```python
from build123d import *

# Parameters (mm, degrees)
BOSS_EXTRUDE1_DEPTH   = 40
BOSS_EXTRUDE1_2_DEPTH = 40
BOSS_EXTRUDE2_DEPTH   = 5


with BuildPart() as part:
    # Sketch2 → Boss-Extrude1 (new body)
    with BuildSketch(Plane.XY.offset(-35)):
        Polygon((-29.235736387, -93.619070837), (-29.235736387, -98.170199329), (-20.059825436, -100.584912737), (-20.059825436, -93.619070837), align=None)
    extrude(amount=BOSS_EXTRUDE1_DEPTH)



with BuildPart() as body_2:
    # Sketch2 → Boss-Extrude1 2 (new body)
    with BuildSketch(Plane.XY.offset(-35)):
        Polygon((29.235736387, -98.170199329), (20.059825436, -100.584912737), (20.059825436, -93.619070837), (29.235736387, -93.619070837), align=None)
    extrude(amount=BOSS_EXTRUDE1_2_DEPTH)


with BuildPart() as part_1:
    add(part.part)

    add(body_2.part)  # Boss-Extrude2 merges body 2
    # Sketch3 → Boss-Extrude2 (add)
    with BuildSketch(Plane.XY):
        Polygon((-46.530024654, -93.619070837), (0.133009642, -93.619070837), (46.530024654, -93.619070837), (46.530024654, -95.999382249), (0.133009642, -107.832641703), (-46.530024654, -95.999382249), align=None)
    extrude(amount=BOSS_EXTRUDE2_DEPTH)


solid = part_1.part
```
Geometry check sheet. Reference: the model listing, model coordinates, mm. A direction names the side the tool comes from. Round coordinates to 2 decimals unless told otherwise and drop trailing zeros. Loops run counter-clockwise (first coordinate to the right, second up) from the corner with the lowest first, then second, coordinate; pieces in that order, holes last. Notation, with made-up numbers: (53.25, 33) - (68.25, 33) arc R29 cw to (68.25, 60) - close; hole circle Ø6 at (73.25, 37). An arc over 180 degrees is marked (long way). Use a Markdown table: item, result.
Q1. Cross-section at A-A on z = -3.5. Record the cut outline in (x, y).
Solutions:
| item | result |
|---|---|
| outline | (-29.24, -98.17) - (-20.06, -100.58) - (-20.06, -93.62) - (-29.24, -93.62) - close; (20.06, -100.58) - (29.24, -98.17) - (29.24, -93.62) - (20.06, -93.62) - close |
Q2. Cross-section at B-B on y = -94.75. Record the cut outline in (x, z).
Solutions:
| item | result |
|---|---|
| outline | (-46.53, 0) - (-29.24, 0) - (-29.24, -35) - (-20.06, -35) - (-20.06, 0) - (20.06, 0) - (20.06, -35) - (29.24, -35) - (29.24, 0) - (46.53, 0) - (46.53, 5) - (-46.53, 5) - close |
Q3. Access from +Z, -Z, +X, -X, +Y, -Y to the whole of each face (thin tool, end or side, straight path). Record for faces 4 (the flat face through (-24.71, -99.36, -17.74)), 5 (the flat face through (-22.87, -102, 2.46)), 6 (the flat face through (29.236, -96, -18)), 7 (the flat face through (-20.06, -97, -18)), 8 (the flat face through (-29.236, -96, -18)).
Solutions:
| item | result |
|---|---|
| face 4 | -Z, -X, -Y |
| face 5 | +Z, -Z, -X, -Y |
| face 6 | -Z, +X, +Y, -Y |
| face 7 | -Z, +Y, -Y |
| face 8 | -Z, -X, +Y, -Y |
Q4. Material ranges on line 1 (X direction, y = -98, z = -22.5); line 2 (Z direction, x = 5.5, y = -104.5); line 3 (Y direction, x = 41, z = 0.5), recorded low to high.
Solutions:
| item | result |
|---|---|
| line 1 | x = -29.24 to -20.06, 20.06 to 29.24 |
| line 2 | z = 0 to 5 |
| line 3 | y = -97.41 to -93.62 |
Q5. Draft check along X on faces 1 (the flat face through (1, -99, 0)), 2 (the flat face through (-46.53, -95, 2)), 3 (the flat face through (24.71, -99.36, -17.74)). Enter one of: released by +X, released by -X, zero draft, split by the parting line, or undercut.
Solutions:
| item | result |
|---|---|
| face 1 | undercut |
| face 2 | released by -X |
| face 3 | released by +X |
Q6. Go/stop test with flat-tipped pins: P1, Ø5, axis at y = -95, z = -20.5, coming from the +X side; P2, Ø5, axis at x = 1, z = -3, coming from the +Y side; P3, Ø7, axis at x = -0.5, y = -101, coming from the -Z side; P4, Ø12, axis at x = 24.5, z = -1, coming from the -Y side. Record where each tip stops, or that it passes through.
Solutions:
| item | result |
|---|---|
| P1 | stops at x = 29.24 |
| P2 | passes through |
| P3 | stops at z = 0 |
| P4 | stops at y = -103.13 |
Q7. Cross-section at C-C on x = -21.5. Record the cut outline in (y, z), plus the area to 3 significant figures.
Solutions:
| item | result |
|---|---|
| outline | (-102.35, 0) - (-100.21, 0) - (-100.21, -35) - (-93.62, -35) - (-93.62, 5) - (-102.35, 5) - close |
| area | 274 mm2 |
Q8. Cross-section at D-D on y = -99.75. Record the cut outline in (x, z), plus the area to 3 significant figures.
Solutions:
| item | result |
|---|---|
| outline | (-31.74, 0) - (-23.23, 0) - (-23.23, -35) - (-20.06, -35) - (-20.06, 0) - (20.06, 0) - (20.06, -35) - (23.23, -35) - (23.23, 0) - (31.82, 0) - (31.82, 5) - (-31.74, 5) - close |
| area | 540 mm2 |
